```python
from build123d import *

# Parameters (mm, degrees)
BOSS_EXTRUDE1_DEPTH = 99.95
SKETCH2_W           = 4
SKETCH2_H           = 19
BOSS_EXTRUDE2_DEPTH = 24.39


with BuildPart() as part:
    # Sketch1 → Boss-Extrude1 (new body)
    with BuildSketch(Plane.XY):
        Polygon((52.648648649, 19.666666667), (56.648648649, 19.666666667), (56.648648649, 38.666666667), (-43.351351351, 38.666666667), (-43.351351351, 19.666666667), (-39.351351351, 19.666666667), (-39.351351351, 34.666666667), (52.648648649, 34.666666667), align=None)
    extrude(amount=BOSS_EXTRUDE1_DEPTH)

    # Sketch2 → Boss-Extrude2 (add)
    with BuildSketch(Plane.XY.offset(99.95)):
        with Locations((-41.351351351, 29.166666667)):
            Rectangle(SKETCH2_W, SKETCH2_H)
        with Locations((54.648648649, 29.166666667)):
            Rectangle(SKETCH2_W, SKETCH2_H)
    extrude(amount=BOSS_EXTRUDE2_DEPTH)


solid = part.part
```
CAD build for the part. Positions are in the model's coordinates, mm. A direction names the side the tool comes from. Round coordinates to 2 decimals unless told otherwise and drop trailing zeros. Order: outer loops, then holes, each group sorted by start corner. A loop starts at its lowest first (then second) coordinate and runs counter-clockwise, first axis right, second up. Notation, with made-up numbers: (15, -39.75) -> (38, -39.75) arc R8 cw to (38, -30.75) -> close; hole circle Ø5 at (59.5, 19.25). An arc over 180 degrees is marked (long way). Write item = value, one per line.
(1) Drill centre lines: L1, parallel to X at y = 26, z = 30; L2, parallel to Y at x = 0.5, z = 40.5; L3, parallel to Z at x = 41, y = 34.75. Where is each one in solid material? Low to high.
Answers follow:
L1 = -43.35 to -39.35, 52.65 to 56.65
L2 = 34.67 to 38.67
L3 = 0 to 99.95
(2) Cut at C-C (z = 67). Write the cut outline in (x, y), plus the area to 3 significant figures.
Answers follow:
outline = (-43.35, 19.67) -> (-39.35, 19.67) -> (-39.35, 34.67) -> (52.65, 34.67) -> (52.65, 19.67) -> (56.65, 19.67) -> (56.65, 38.67) -> (-43.35, 38.67) -> close
area = 520 mm²
(3) Flat gauge pins, fed straight in: P1, Ø12, axis at x = -26, z = 20.5, coming from the -Y side; P2, Ø1.2, axis at x = -2, y = 36, coming from the +Z side. Where does each tip first touch, or does it go through?
Answers follow:
P1 = 34.67
P2 = 99.95
(4) Cut at B-B (z = 116). Write the cut outline in (x, y).
Answers follow:
outline = (-43.35, 19.67) -> (-39.35, 19.67) -> (-39.35, 38.67) -> (-43.35, 38.67) -> close; (52.65, 19.67) -> (56.65, 19.67) -> (56.65, 38.67) -> (52.65, 38.67) -> close
(5) Pull direction X, two halves, no side cores. Call faces 1 (the flat face through (56.649, 29, 61)), 2 (the flat face through (6, 37, 99.95)), 3 (the flat face through (-43.351, 29, 61)), 4 (the flat face through (-41, 29, 124.34)): +X half, -X half, draft (parallel to the pull), parting line (faces both ways), or undercut.
Answers follow:
face_1 = +X half
face_2 = undercut
face_3 = -X half
face_4 = draft
(6) 3-axis set-ups, long thin cutter, end or side, ignore diameter. For faces 5 (the flat face through (6, 34.667, 49)), 6 (the flat face through (55, 29, 124.34)): which of +Z, -Z, +X, -X, +Y, -Y reach the whole face in a straight line?
Answers follow:
face_5 = +Z, -Z, -Y
face_6 = +Z, +X, -X, +Y, -Y
(7) Cut at A-A (y = 31). Write the cut outline in (x, z).
Answers follow:
outline = (-43.35, 0) -> (-39.35, 0) -> (-39.35, 124.34) -> (-43.35, 124.34) -> close; (52.65, 0) -> (56.65, 0) -> (56.65, 124.34) -> (52.65, 124.34) -> close
(8) Cut at D-D (x = -24.5). Write the cut outline in (y, z), plus the area to 3 significant figures.
Answers follow:
outline = (34.67, 0) -> (38.67, 0) -> (38.67, 99.95) -> (34.67, 99.95) -> close
area = 400 mm²
